```python
from build123d import *

# Parameters (mm, degrees)
SKETCH1_R           = 2.75
BOSS_EXTRUDE1_DEPTH = 30
SKETCH2_W           = 10
SKETCH2_H           = 6
CUT_EXTRUDE1_DEPTH  = 55
CUT_EXTRUDE2_DEPTH  = 17


with BuildPart() as part:
    # Sketch1 → Boss-Extrude1 (new body)
    with BuildSketch(Plane(origin=(0, 0, 0), x_dir=(1, 0, 0), z_dir=(0, 1, 0))):
        with BuildLine():
            Line((7.5, 12.990381057), (7.5, 75))
            ThreePointArc((7.5, 75), (0, 82.5), (-7.5, 75))
            Line((-7.5, 75), (-7.5, 12.990381057))
            ThreePointArc((-7.5, 12.990381057), (-13.858192988, -5.740251485), (3.882285677, -14.488887394))
            Line((3.882285677, -14.488887394), (17.67766953, -28.284271247))
            ThreePointArc((17.67766953, -28.284271247), (28.284271247, -28.284271247), (28.284271247, -17.67766953))
            Line((28.284271247, -17.67766953), (14.488887394, -3.882285677))
            ThreePointArc((14.488887394, -3.882285677), (13.858192988, 5.740251485), (7.5, 12.990381057))
        make_face()
        Circle(SKETCH1_R, mode=Mode.SUBTRACT)
        with Locations((22.980970389, -22.980970389)):
            Circle(SKETCH1_R, mode=Mode.SUBTRACT)
        with Locations((0, 75)):
            Circle(SKETCH1_R, mode=Mode.SUBTRACT)
    extrude(amount=BOSS_EXTRUDE1_DEPTH)

    # Sketch2 → Cut-Extrude1 (cut)
    with BuildSketch(Plane(origin=(7.5, 0, 0), x_dir=(0, 0, -1), z_dir=(1, 0, 0))):
        Polygon((75, 30), (75, 24), (88.340353556, 24), (88.340353556, 42.222756781), (65, 42.222756781), (65, 30), align=None)
        Polygon((88.340353556, 6), (75, 6), (75, 0), (65, 0), (65, -8.682673162), (88.340353556, -8.682673162), align=None)
        with Locations((70, 3)):
            Rectangle(SKETCH2_W, SKETCH2_H)
        with Locations((70, 27)):
            Rectangle(SKETCH2_W, SKETCH2_H)
    extrude(amount=-CUT_EXTRUDE1_DEPTH, mode=Mode.SUBTRACT)

    # Sketch3 → Cut-Extrude2 (cut)
    with BuildSketch(Plane(origin=(5.303300859, 0, -5.303300859), x_dir=(-0.707106781, 0, -0.707106781), z_dir=(0.707106781, 0, -0.707106781))):
        Polygon((-32.5, 21), (-32.5, 15), (-32.5, 9), (-22.5, 9), (-22.5, 21), align=None)
        Polygon((-32.5, 9), (-32.5, 15), (-32.5, 21), (-50.580242044, 21), (-50.580242044, 9), align=None)
    extrude(amount=-CUT_EXTRUDE2_DEPTH, mode=Mode.SUBTRACT)


solid = part.part
```
Geometry: final body of the model. Coordinates: model frame, mm. A direction names the side the tool comes from. Give positions to 0.01 mm unless a question says otherwise; leave off trailing zeros. Order: outer loops, then holes, each group sorted by start corner. A loop starts at its lowest first (then second) coordinate and runs counter-clockwise, first axis right, second up. Notation, with made-up numbers: (28.25, -22) -> (39.25, -22) arc R20 ccw to (39.25, -15) -> close; hole circle Ø1 at (75, 26). An arc over 180 degrees is marked (long way). Write each question's results on one line, items separated by ' | '. Start each with the question number.
1) Section D-D (x = 12.5). Return loops of the section in (y, z), then the cut area to 3 significant figures.
2) Line query: line 1 (Z direction, x = 0, y = 14.25); line 2 (X direction, y = 17, z = 0); line 3 (X direction, y = 15, z = -19). Output: solid intervals per line, ascending. Write a range as from..to.
3) Draft query along Y for faces 1 (the flat face through (0, 6, -72)), 2 (the flat face through (15.98, 14.92, 15.84)), 3 (the cylindrical face through (-13.97, 14.79, 5.46)). Return one class per face: pulls with the +Y half, pulls with the -Y half, needs draft (parallel to the pull), parting line crosses it, or undercut.
4) Section C-C (y = 26.25). Return loops of the section in (x, z), then the cut area to 3 significant figures.
5) First-contact query: pin 1 (15 mm diameter, centred on y = 19, z = -52.5, fed in from -X); pin 2 (4 mm diameter, centred on y = 5, z = -60.5, fed in from +X); pin 3 (3 mm diameter, centred on x = -1, y = 2.5, fed in from -Z). Flat tips, straight axial feed; report the tip coordinate or a pass-through.
6) Section B-B (z = 0). Return loops of the section in (x, y).
7) Section A-A (x = 0). Return loops of the section in (y, z).
8) Set-up query: faces 4 (the flat face through (7.5, 15, -44)), 5 (the flat face through (20.7, 21, 20.6)), 6 (the flat face through (0, 27, -65)). Return all of +Z, -Z, +X, -X, +Y, -Y with unobstructed straight access to the full face (end or side cutting, diameter ignored); none if empty.
Calculated:
1) outline: (0, -8.29) -> (30, -8.29) -> (30, 23.11) -> (21, 23.11) -> (21, 19.32) -> (9, 19.32) -> (9, 23.11) -> (0, 23.11) -> close | area: 897 mm2
2) line 1: -82.5..-77.75, -72.25..-2.75, 2.75..15 | line 2: -15..-2.75, 2.75..15 | line 3: -7.5..7.5
3) face 1: pulls with the -Y half | face 2: undercut | face 3: needs draft
4) outline: (-7.5, -65) -> (7.5, -65) -> (7.5, -12.99) arc R15 ccw to (14.49, 3.88) -> (28.28, 17.68) arc R7.5 ccw to (17.68, 28.28) -> (3.88, 14.49) arc R15 ccw to (-7.5, -12.99) -> close; hole circle Ø5.5 at (0, 0); hole circle Ø5.5 at (22.98, 22.98) | area: 1,780 mm2
5) pin 1: x = -7.5 | pin 2: x = 7.5 | pin 3: z = -65
6) outline: (-15, 0) -> (-2.75, 0) -> (-2.75, 30) -> (-15, 30) -> close; (2.75, 0) -> (15, 0) -> (15, 30) -> (2.75, 30) -> close
7) outline: (0, -65) -> (6, -65) -> (6, -72.25) -> (24, -72.25) -> (24, -65) -> (30, -65) -> (30, -2.75) -> (0, -2.75) -> close; (0, 2.75) -> (30, 2.75) -> (30, 15) -> (0, 15) -> close; (6, -82.5) -> (24, -82.5) -> (24, -77.75) -> (6, -77.75) -> close
8) face 4: -Z, +X, +Y, -Y | face 5: +Z, +X | face 6: -Z, +X, -X, +Y
